from build123d import *

# Parameters (mm, degrees)
F3_DEPTH = 3
F4_R     = 0.5


with BuildPart() as f1:
    # F0 (on Front) → F1 (revolve)
    with BuildSketch(Plane.XZ):
        Polygon((-3, -30), (0, -30), (0, 6), (-5, 6), (-5, 0), (-3, 0), align=None)
    revolve(axis=Axis((0, 0, -12), (0, 0, -1)))

    # F2 (on face) → F3 (cut)
    with BuildSketch(Plane.XY.offset(6)):
        Polygon((1.443376, 2.5), (-1.443376, 2.5), (-2.886751, 0), (-1.443376, -2.5), (1.443376, -2.5), (2.886751, 0), align=None)
    extrude(amount=-F3_DEPTH, mode=Mode.SUBTRACT)

    # F4
    f4_edges = [f1.edges().sort_by_distance(p)[0] for p in [
        (5, 0, 6),
    ]]
    fillet(f4_edges, radius=F4_R)


solid = f1.part
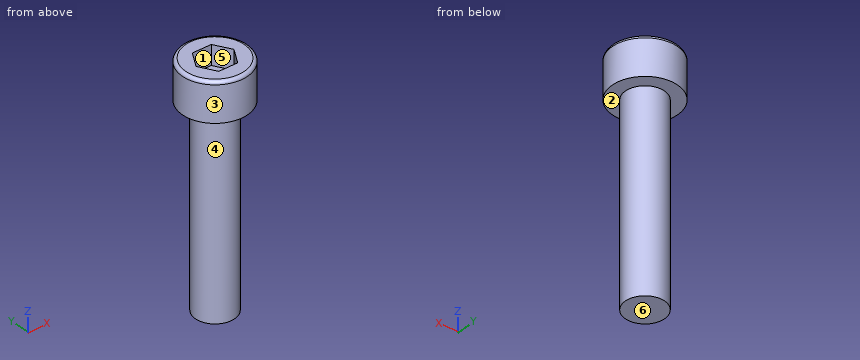
For this review, take the finished solid that the model builds, in its own axes (mm). Face numbers are marked on the shaded views. A direction names the side the tool comes from. Give positions to 0.01 mm unless a question says otherwise; leave off trailing zeros. Loops run counter-clockwise (first coordinate to the right, second up) from the corner with the lowest first, then second, coordinate; pieces in that order, holes last. Notation, with made-up numbers: (-9, 40) -> (48, 40) arc R17 cw to (48, 65) -> close; hole circle Ø11 at (8, -8.75). An arc over 180 degrees is marked (long way). One line per question, with ' | ' between items.
1) The part is to be moulded in two halves that separate along Y. For the marked faces 4, 5 and 6, say which applies: +Y half, -Y half, draft (parallel to the pull), parting line (faces both ways), or undercut.
Resolved:
face 4: parting line | face 5: undercut | face 6: draft
2) For the marked faces 1, 2 and 3, list the 3-axis set-ups (+Z, -Z, +X, -X, +Y, -Y) from which the entire face can be reached by the end or side of a thin tool; tool diameter is ignored.
Resolved:
face 1: +Z | face 2: -Z | face 3: +Z, -Z
3) Insertion check: pin 1 Ø6 at (y, z) = (-3, -18) entering from -X; pin 2 Ø1 at (x, z) = (0, -16) entering from -Y; pin 3 Ø2.5 at (x, y) = (0, 0.5) entering from +Z. Each pin has a flat end and moves straight along its axis. Give the tip position at first contact, or say it passes through.
Resolved:
pin 1: stops at x = -3 | pin 2: stops at y = -3 | pin 3: stops at z = 3
4) To check wall thickness, follow probe 1 along Z at (x, y) = (-3.5, 0.5); probe 2 along Z at (x, y) = (-0.25, 0.5); probe 3 along Y at (x, z) = (-1.5, -1.5). State the ranges of each line that lie inside material, in increasing order.
Resolved:
probe 1: z = 0 to 6 | probe 2: z = -30 to 3 | probe 3: y = -2.6 to 2.6
5) We need section B-B (z = -15.5). Write out the cut boundary in (x, y).
Resolved:
outline: circle Ø6 at (0, 0)
6) We need section A-A (x = 0). Write out the cut boundary in (y, z).
Resolved:
outline: (-5, 0) -> (-3, 0) -> (-3, -30) -> (3, -30) -> (3, 0) -> (5, 0) -> (5, 5.5) arc R0.5 ccw to (4.5, 6) -> (2.5, 6) -> (2.5, 3) -> (-2.5, 3) -> (-2.5, 6) -> (-4.5, 6) arc R0.5 ccw to (-5, 5.5) -> close
